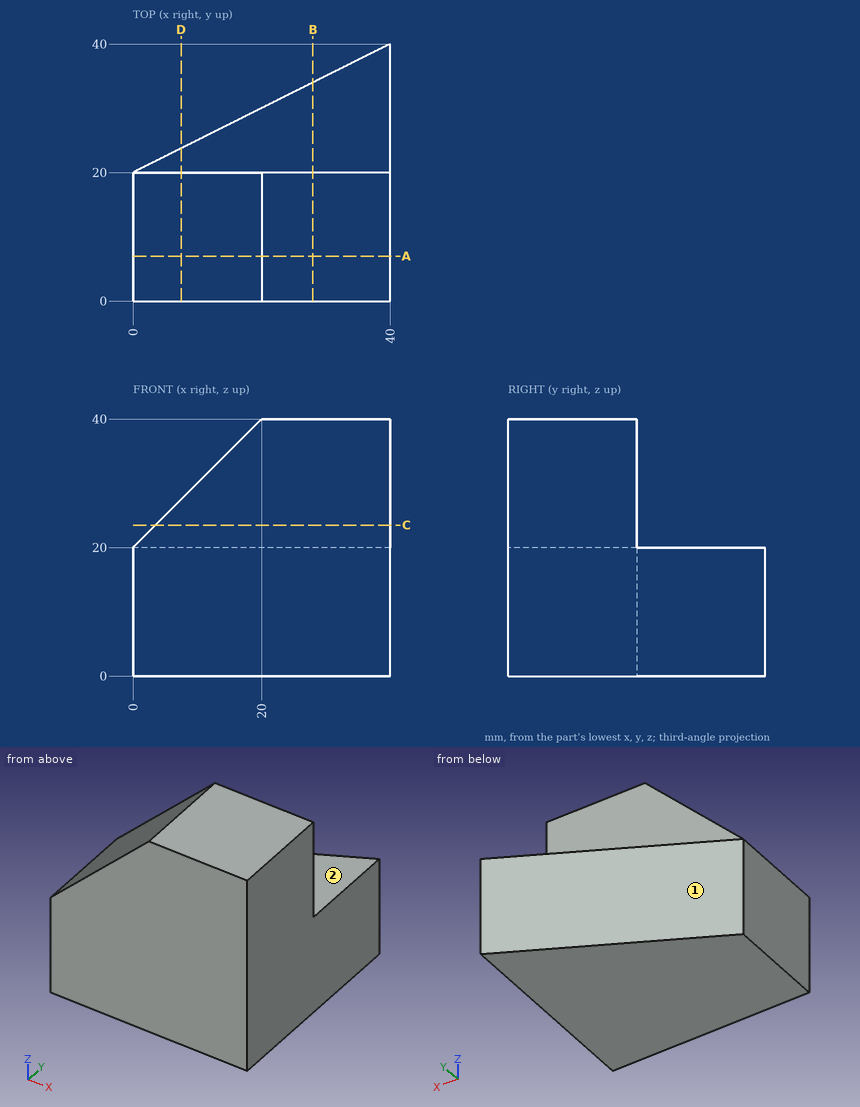
Could you check a few things on this drawing? It's one solid part, dimensions in mm from its lowest x, y, z. A direction names the side the tool comes from. Give positions to 0.01 mm unless a question says otherwise; leave off trailing zeros. Order: outer loops, then holes, each group sorted by start corner. A loop starts at its lowest first (then second) coordinate and runs counter-clockwise, first axis right, second up. Notation, with made-up numbers: (62.5, 85) - (105.5, 85) arc R19 cw to (105.5, 99) - close; hole circle Ø4 at (12.25, 78). An arc over 180 degrees is marked (long way). One line per item, written item: value. Start each with the question number.
1. If I drill on probe 1 along Y at (x, z) = (36.5, 36); probe 2 along X at (y, z) = (3.5, 33.5), over which ranges is the centre line in solid material (lowest first)?
2. For P1, Ø6, axis at x = 18, z = 26.5, coming from the +Y side; P2, Ø8, axis at x = 17, y = 34, coming from the -Z side; P3, Ø5, axis at x = 10.5, z = 12, coming from the +Y side; P4, Ø10, axis at y = 27, z = 6, coming from the -X side, each with a flat end and sliding along its axis, tell me the tip position at first contact or that it passes through.
3. For the marked faces 1 and 2, which set-ups out of +Z, -Z, +X, -X, +Y, -Y let a thin tool reach every point of the face, with its end or its side?
4. Imagine slicing it at B-B on x = 28. List the corners of the cut face in (y, z) for me.
5. Imagine slicing it at A-A on y = 7. List the corners of the cut face in (x, z) for me, plus the area to 3 significant figures.
6. Imagine slicing it at C-C on z = 23.5. List the corners of the cut face in (x, y) for me, plus the area to 3 significant figures.
7. Imagine slicing it at D-D on x = 7.5. List the corners of the cut face in (y, z) for me, plus the area to 3 significant figures.
Values:
1. probe 1: 0 to 20
1. probe 2: 13.5 to 40
2. P1: y = 20
2. P2: through
2. P3: y = 26.5
2. P4: x = 4
3. face 1: +Z, -Z, -X, +Y
3. face 2: +Z, +X, -X, +Y
4. outline: (0, 0) - (34, 0) - (34, 20) - (20, 20) - (20, 40) - (0, 40) - close
5. outline: (0, 0) - (40, 0) - (40, 40) - (20, 40) - (0, 20) - close
5. area: 1,400 mm²
6. outline: (3.5, 0) - (40, 0) - (40, 20) - (3.5, 20) - close
6. area: 730 mm²
7. outline: (0, 0) - (23.75, 0) - (23.75, 20) - (20, 20) - (20, 27.5) - (0, 27.5) - close
7. area: 625 mm²
